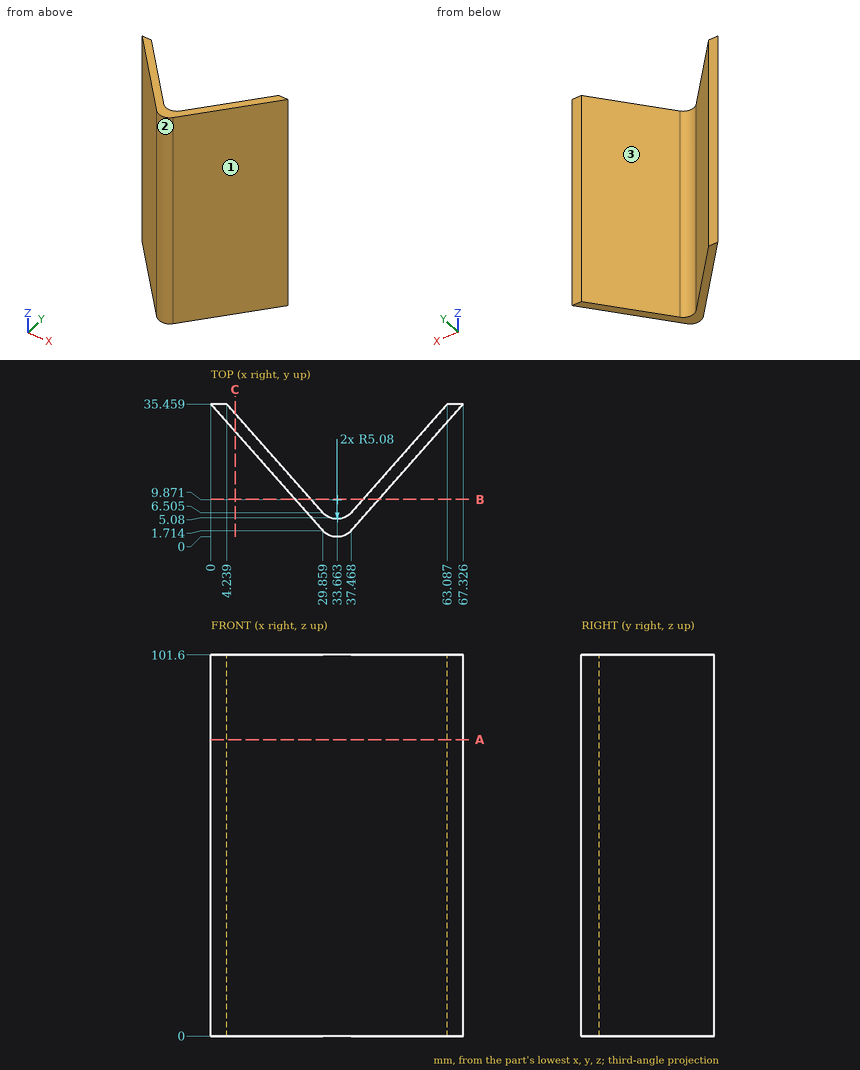
Verification items for this drawing (mm, ordinates from the low corner). Give positions to 0.01 mm unless a question says otherwise; leave off trailing zeros. Write each loop counter-clockwise with the first axis right and the second up, starting at its lowest first coordinate (ties: lowest second). Pieces come first, ordered by that corner, then holes. Notation, with made-up numbers: (68, 44) - (94, 44) arc R30 ccw to (94, 77) - close; hole circle Ø11 at (22.5, -33.75). An arc over 180 degrees is marked (long way). Answer as CSV lines item,"result". Start each with the question number.
1. Thickness scan on line 1 (X direction, y = 19, z = 64) (1 decimal); line 2 (X direction, y = 13, z = 66) (1 decimal); line 3 (Y direction, x = 33, z = 56) (1 decimal). Record the ranges inside material, lowest first.
2. Depth check by flat-ended pin: pin 1 (1 mm diameter, centred on y = 24.5, z = 87.5, fed in from -X) (1 decimal); pin 2 (3 mm diameter, centred on x = 13.5, z = 41.5, fed in from +Y); pin 3 (1 mm diameter, centred on x = 17.5, z = 17, fed in from +Y); pin 4 (6 mm diameter, centred on x = 50.5, y = 21.5, fed in from +Z). Enter the tip coordinate at first touch or a pass-through.
3. Sectioned sample at A-A (z = 79). Record the boundary of the cut face in (x, y) (1 decimal).
4. Draft check along X on the marked faces 1, 2 and 3. Enter one of: pulls with the +X half, pulls with the -X half, needs draft (parallel to the pull), parting line crosses it, or undercut.
5. Sectioned sample at C-C (x = 6.5). Record the boundary of the cut face in (y, z) (1 decimal), then the cut area to 3 significant figures.
6. Sectioned sample at B-B (y = 10). Record the boundary of the cut face in (x, z).
Derived:
1,line 1,"14.6 to 18.8, 48.5 to 52.8"
1,line 2,"19.9 to 24.1, 43.2 to 47.5"
1,line 3,"0 to 4.8"
2,pin 1,"x = 9.3"
2,pin 2,"y = 26.69"
2,pin 3,"y = 21.04"
2,pin 4,"z = 101.6"
3,outline,"(0, 35.5) - (29.9, 1.7) arc R5.1 ccw to (37.5, 1.7) - (67.3, 35.5) - (63.1, 35.5) - (37.5, 6.5) arc R5.1 cw to (29.9, 6.5) - (4.2, 35.5) - close"
4,face 1,"pulls with the +X half"
4,face 2,"parting line crosses it"
4,face 3,"undercut"
5,outline,"(28.1, 0) - (32.9, 0) - (32.9, 101.6) - (28.1, 101.6) - close"
5,area,"487 mm²"
6,outline,"(22.53, 0) - (26.77, 0) - (26.77, 101.6) - (22.53, 101.6) - close; (40.56, 0) - (44.8, 0) - (44.8, 101.6) - (40.56, 101.6) - close"
